from build123d import *

# Parameters (mm, degrees)
SKETCH1_R               = 4
SKETCH1_R_2             = 5
BOSS_EXTRUDE1_DEPTH     = 17
SKETCH1_3_R             = 4
BOSS_EXTRUDE2_DEPTH     = 54
SKETCH2_R               = 1.5
CUT_EXTRUDE1_DEPTH      = 6
CUT_EXTRUDE1_DEPTH_BACK = 6


with BuildPart() as part:
    # Sketch1 → Boss-Extrude1 (new body)
    with BuildSketch(Plane(origin=(0, 0, 0), x_dir=(1, 0, 0), z_dir=(0, 1, 0))):
        Circle(SKETCH1_R)
        Circle(SKETCH1_R_2)
        Circle(SKETCH1_R, mode=Mode.SUBTRACT)
    extrude(amount=BOSS_EXTRUDE1_DEPTH)

    # Sketch1<3> → Boss-Extrude2 (add)
    with BuildSketch(Plane(origin=(0, 0, 0), x_dir=(1, 0, 0), z_dir=(0, 1, 0))):
        Circle(SKETCH1_3_R)
    extrude(amount=BOSS_EXTRUDE2_DEPTH)

    # Sketch2 → Cut-Extrude1 (cut, two sides)
    with BuildSketch(Plane.XY) as cut_extrude1_sk:
        with Locations((0, 50)):
            Circle(SKETCH2_R)
        with Locations((0, 4)):
            Circle(SKETCH2_R)
    extrude(amount=CUT_EXTRUDE1_DEPTH, mode=Mode.SUBTRACT)
    extrude(cut_extrude1_sk.sketch, amount=-CUT_EXTRUDE1_DEPTH_BACK, mode=Mode.SUBTRACT)


solid = part.part
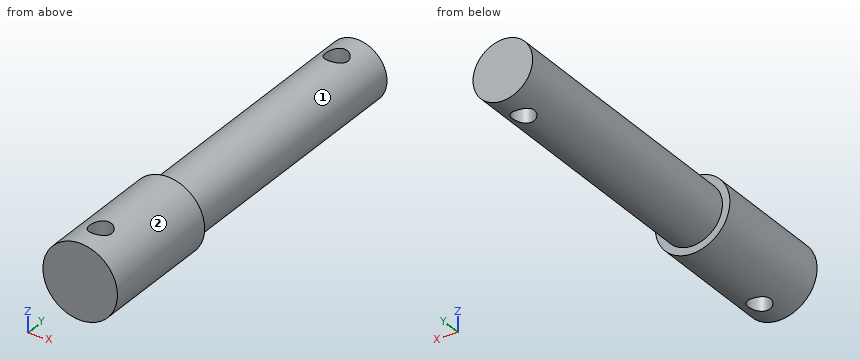
Geometry check sheet. Reference: the model listing, model coordinates, mm. Face numbers are marked on the shaded views. A direction names the side the tool comes from. Give positions to 0.01 mm unless a question says otherwise; leave off trailing zeros. Loops run counter-clockwise (first coordinate to the right, second up) from the corner with the lowest first, then second, coordinate; pieces in that order, holes last. Notation, with made-up numbers: (-31.75, 88) -> (14.25, 88) arc R24 ccw to (14.25, 112) -> close; hole circle Ø4 at (-40, 25.5). An arc over 180 degrees is marked (long way). Answer in a Markdown table with one row per item. Add a question column.
1) Set-up check for the marked faces 1 and 2: record each of +Z, -Z, +X, -X, +Y, -Y from which the full face is reachable in a straight line by a thin tool's end or side.
2) Cross-section at D-D on x = -3.25. Record the boundary of the cut face in (y, z).
3) Cross-section at A-A on x = 0. Record the boundary of the cut face in (y, z).
4) Cross-section at C-C on y = 4. Record the boundary of the cut face in (x, z), and give its area (3 significant figures).
5) Material ranges on probe 1 along Y at (x, z) = (0, -0.5); probe 2 along Y at (x, z) = (-3, 3.25); probe 3 along X at (y, z) = (4, -2.5), recorded low to high. Write a range as from..to.
6) Gauge pin test, flat ends, axial feed: P1, Ø2, axis at x = -1.5, z = 0.5, coming from the -Y side; P2, Ø6, axis at x = -2, y = 38.5, coming from the -Z side; P3, Ø6, axis at x = 2.5, y = 23.5, coming from the +Z side; P4, Ø1.8, axis at x = 0, y = 4, coming from the +Z side. Record the tip position at first contact, or that the pin passes through.
7) Cross-section at B-B on z = 0. Record the boundary of the cut face in (x, y), and give its area (3 significant figures).
Outcome:
| question | item | result |
|---|---|---|
| 1 | face 1 | +Y |
| 1 | face 2 | +Y, -Y |
| 2 | outline | (0, -3.8) -> (17, -3.8) -> (17, -2.33) -> (54, -2.33) -> (54, 2.33) -> (17, 2.33) -> (17, 3.8) -> (0, 3.8) -> close |
| 3 | outline | (0, -5) -> (2.5, -5) -> (2.5, 5) -> (0, 5) -> close; (5.5, -5) -> (17, -5) -> (17, -4) -> (48.5, -4) -> (48.5, 4) -> (17, 4) -> (17, 5) -> (5.5, 5) -> close; (51.5, -4) -> (54, -4) -> (54, 4) -> (51.5, 4) -> close |
| 4 | outline | (-1.5, -4.77) -> (-1.5, 4.77) arc R5 ccw to start; (1.5, -4.77) arc R5 ccw to (1.5, 4.77) -> close |
| 4 | area | 49.0 mm^2 |
| 5 | probe 1 | y = 0..2.5, 5.5..48.5, 51.5..54 |
| 5 | probe 2 | y = 0..17 |
| 5 | probe 3 | x = -4.33..-1.5, 1.5..4.33 |
| 6 | P1 | stops at y = 0 |
| 6 | P2 | stops at z = -4 |
| 6 | P3 | stops at z = 4 |
| 6 | P4 | passes through |
| 7 | outline | (-5, 0) -> (5, 0) -> (5, 17) -> (4, 17) -> (4, 54) -> (-4, 54) -> (-4, 17) -> (-5, 17) -> close; hole circle Ø3 at (0, 4); hole circle Ø3 at (0, 50) |
| 7 | area | 452 mm^2 |
